Read the model definition and answer for the solid it produces. Units are mm, in the model's axes. Face numbers are marked on the shaded views. A direction names the side the tool comes from. Give positions to 0.01 mm unless a question says otherwise; leave off trailing zeros. Write each loop counter-clockwise with the first axis right and the second up, starting at its lowest first coordinate (ties: lowest second). Pieces come first, ordered by that corner, then holes. Notation, with made-up numbers: M 46.25,15 L 77.25,15 A10 ccw 77.25,20 Z; hole C -39,1.25 d4. An arc over 180 degrees is marked long. Use a Markdown table: item, result. Add a question column.
Item 1: A cutting plane is placed at D-D on z = 2. Determine the outline of the cut face in (x, y).
Item 2: A cutting plane is placed at C-C on z = 7. Determine the outline of the cut face in (x, y).
Item 3: A cutting plane is placed at B-B on y = 0. Determine the outline of the cut face in (x, z), then the cut area to 4 significant figures.
Item 4: Consider probe 1 along Y at (x, z) = (0, 9.2); probe 2 along Y at (x, z) = (4.65, 2); probe 3 along Z at (x, y) = (-3, -0.25). Determine where each line is inside the solid, lowest interval first. Write a range as [from, to].
Item 5: For the marked faces 4, 5 and 6, determine the directions among +Z, -Z, +X, -X, +Y, -Y from which every point of the face is accessible in a straight line to the end or side of a thin tool.
Item 6: A cutting plane is placed at A-A on x = 0. Determine the outline of the cut face in (y, z).
Item 7: The mould has two halves that part along Y. Classify the marked faces 1, 2 and 3: pulls with the +Y half, pulls with the -Y half, needs draft (parallel to the pull), parting line crosses it, or undercut.
Item 8: Given P1, Ø1.5, axis at y = -1.5, z = 8.5, coming from the -X side; P2, Ø2.5, axis at x = 1, y = 0, coming from the -Z side; P3, Ø3, axis at y = -1, z = 8.5, coming from the -X side, each flat-ended and moving along its own axis, determine where each tip first touches the part or whether it passes through.
from build123d import *

# Parameters (mm, degrees)
CONNECTOR_M5X0_8_TAPPED_HOLE_D        = 4.2
SET_SCREW_1_M3X0_5_TAPPED_HOLE_REACH  = 16.767
SET_SCREW_1_M3X0_5_TAPPED_HOLE_BORE_R = 1.25
SET_SCREW_2_PATTERN_COUNT             = 2


with BuildPart() as part:
    # Body Sketch → Body Revolve (revolve)
    with BuildSketch(Plane(origin=(0, 0, 0), x_dir=(-1, 0, 0), z_dir=(0, 1, 0))):
        Polygon((1, 10.5), (3.7, 10.5), (3.7, 5.5), (5.4, 4), (5.4, 0), (2.5, 0), (2.5, 5), (1, 5), align=None)
    revolve(axis=Axis((0, 0, 0), (0, 0, 1)))

    # Connector M5x0.8 Tapped Hole (through all)
    with Locations(Plane.XY.offset(10.5)):
        with Locations((0, 0)):
            Hole(CONNECTOR_M5X0_8_TAPPED_HOLE_D / 2)

    # Set Screw 1 M3x0.5 Tapped Hole bore (on position points) → Set Screw 1 M3x0.5 Tapped Hole (cut, up to next)
    with BuildSketch(Plane(origin=(5.4, 0, 2), x_dir=(0, 1, 0), z_dir=(1, 0, 0)), mode=Mode.PRIVATE) as set_screw_1_m3x0_5_tapped_hole_sk1:
        Circle(SET_SCREW_1_M3X0_5_TAPPED_HOLE_BORE_R)
    set_screw_1_m3x0_5_tapped_hole_tool1 = extrude(set_screw_1_m3x0_5_tapped_hole_sk1.sketch, amount=-SET_SCREW_1_M3X0_5_TAPPED_HOLE_REACH, mode=Mode.PRIVATE) & part.part
    set_screw_1_m3x0_5_tapped_hole = set_screw_1_m3x0_5_tapped_hole_tool1.solids().sort_by_distance((5.4, 0, 2))[0]
    add(set_screw_1_m3x0_5_tapped_hole, mode=Mode.SUBTRACT)

    # Set Screw 2 Pattern: Set Screw 1 M3x0.5 Tapped Hole ×2 about axis
    set_screw_2_pattern_axis = Axis((0, 0, 0), (0, 0, 1))
    for i in range(1, SET_SCREW_2_PATTERN_COUNT):
        add(set_screw_1_m3x0_5_tapped_hole.rotate(set_screw_2_pattern_axis, i * 360 / SET_SCREW_2_PATTERN_COUNT), mode=Mode.SUBTRACT)


solid = part.part
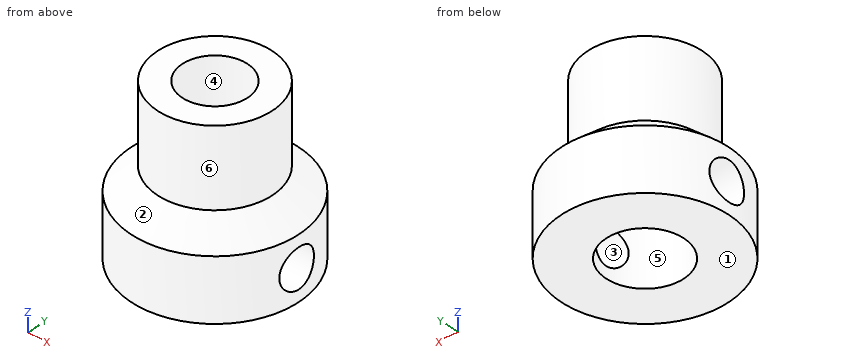
Filled in:
| question | item | result |
|---|---|---|
| 1 | outline | M -5.25,-1.25 A5.4 ccw 5.25,-1.25 L 2.17,-1.25 A2.5 cw -2.17,-1.25 Z; M -5.25,1.25 L -2.17,1.25 A2.5 cw 2.17,1.25 L 5.25,1.25 A5.4 ccw Z |
| 2 | outline | C 0,0 d7.4; hole C 0,0 d4.2 |
| 3 | outline | M -5.4,0 L -2.5,0 L -2.5,0.75 L -5.4,0.75 Z; M -5.4,3.25 L -2.5,3.25 L -2.5,5 L -2.1,5 L -2.1,10.5 L -3.7,10.5 L -3.7,5.5 L -5.4,4 Z; M 2.1,5 L 2.5,5 L 2.5,3.25 L 5.4,3.25 L 5.4,4 L 3.7,5.5 L 3.7,10.5 L 2.1,10.5 Z; M 2.5,0 L 5.4,0 L 5.4,0.75 L 2.5,0.75 Z |
| 3 | area | 31.25 mm² |
| 4 | probe 1 | [-3.7, -2.1], [2.1, 3.7] |
| 4 | probe 2 | [-2.75, -1.25], [1.25, 2.75] |
| 4 | probe 3 | [0, 0.78], [3.22, 10.5] |
| 5 | face 4 | +Z, -Z |
| 5 | face 5 | -Z |
| 5 | face 6 | +Z |
| 6 | outline | M -5.4,0 L -2.5,0 L -2.5,5 L -2.1,5 L -2.1,10.5 L -3.7,10.5 L -3.7,5.5 L -5.4,4 Z; M 2.1,5 L 2.5,5 L 2.5,0 L 5.4,0 L 5.4,4 L 3.7,5.5 L 3.7,10.5 L 2.1,10.5 Z |
| 7 | face 1 | needs draft |
| 7 | face 2 | parting line crosses it |
| 7 | face 3 | undercut |
| 8 | P1 | x = -3.62 |
| 8 | P2 | z = 5 |
| 8 | P3 | x = -3.7 |
